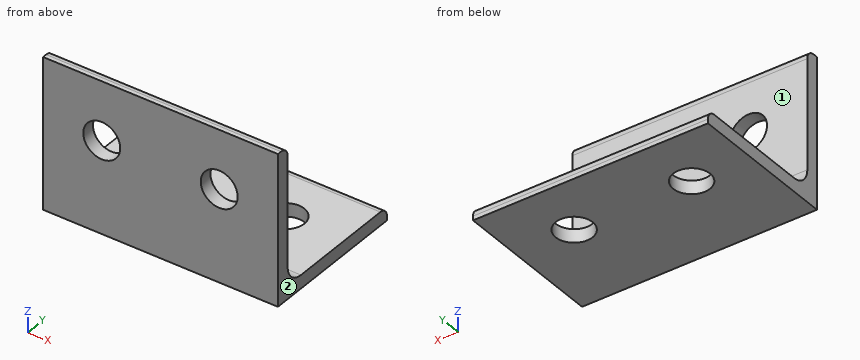
```python
from build123d import *

# Parameters (mm, degrees)
ANGLES_EQUAL_90_X_90_X_8_1_DEPTH = 140
SKETCH12_R                       = 11
CUT_EXTRUDE1_DEPTH               = 190.208879284
LPATTERN1_COUNT                  = 2
LPATTERN1_PITCH                  = 70
CIRPATTERN4_COUNT                = 2
CIRPATTERN4_ANGLE                = 90
CIRPATTERN4_COPY_1_SKETCH_R      = 11
CIRPATTERN4_COPY_1_DEPTH         = 190.208879284


with BuildPart() as part:
    # Sketch11 → Angles equal 90 X 90 X 8(1) (new body)
    with BuildSketch(Plane(origin=(0, 45, 45), x_dir=(0, 1, 0), z_dir=(1, 0, 0))):
        with BuildLine():
            Line((-45, 45), (-45, -45))
            Line((-45, -45), (45, -45))
            Line((45, -45), (45, -42.5))
            ThreePointArc((45, -42.5), (43.389087297, -38.610912703), (39.5, -37))
            Line((39.5, -37), (-26, -37))
            ThreePointArc((-26, -37), (-33.778174593, -33.778174593), (-37, -26))
            Line((-37, -26), (-37, 39.5))
            ThreePointArc((-37, 39.5), (-38.610912703, 43.389087297), (-42.5, 45))
            Line((-42.5, 45), (-45, 45))
        make_face()
    extrude(amount=ANGLES_EQUAL_90_X_90_X_8_1_DEPTH)

    # Sketch12 → Cut-Extrude1 (cut, symmetric)
    with BuildSketch(Plane(origin=(0, 0, 0), x_dir=(1, 0, 0), z_dir=(0, 1, 0))):
        with Locations(Location((35, -55, 0), (0, 0, 90))):
            Circle(SKETCH12_R)
    cut_extrude1 = extrude(amount=CUT_EXTRUDE1_DEPTH, both=True, mode=Mode.SUBTRACT)

    # LPattern1: Cut-Extrude1 ×2
    with Locations(*[(i * LPATTERN1_PITCH, 0, 0) for i in range(1, LPATTERN1_COUNT)]):
        add(cut_extrude1, mode=Mode.SUBTRACT)

    # CirPattern4: Cut-Extrude1 ×2 about axis
    cirpattern4_axis = Axis((-18.99, 0, 0), (-1, 0, 0))
    for i in range(1, CIRPATTERN4_COUNT):
        add(cut_extrude1.rotate(cirpattern4_axis, i * CIRPATTERN4_ANGLE / (CIRPATTERN4_COUNT - 1)), mode=Mode.SUBTRACT)

    # CirPattern4 copy 1 sketch → CirPattern4 copy 1 (cut, symmetric)
    with BuildSketch(Plane(origin=(70, 0, 0), x_dir=(1, 0, 0), z_dir=(0, 0, -1))):
        with Locations(Location((35, -55, 0), (0, 0, 90))):
            Circle(CIRPATTERN4_COPY_1_SKETCH_R)
    extrude(amount=CIRPATTERN4_COPY_1_DEPTH, both=True, mode=Mode.SUBTRACT)


solid = part.part
```
CAD build for the part. Positions are in the model's coordinates, mm. Face numbers are marked on the shaded views. A direction names the side the tool comes from. Round coordinates to 2 decimals unless told otherwise and drop trailing zeros. Order: outer loops, then holes, each group sorted by start corner. A loop starts at its lowest first (then second) coordinate and runs counter-clockwise, first axis right, second up. Notation, with made-up numbers: (-32, 33) - (16, 33) arc R4 ccw to (16, 40) - close; hole circle Ø6 at (73.25, -31.75). An arc over 180 degrees is marked (long way). Answer in a Markdown table with one row per item. Add a question column.
(1) Band-saw the part on B-B on z = 55. List the corners of the cut face in (x, y), and give its area (3 significant figures).
(2) Band-saw the part on D-D on x = 52.5. List the corners of the cut face in (y, z), and give its area (3 significant figures).
(3) Drop flat-ended pins along their axis: pin 1 Ø19.5 at (x, z) = (72.5, 46) entering from +Y; pin 2 Ø1.5 at (x, y) = (52, 38) entering from +Z; pin 3 Ø5 at (x, z) = (125.5, 26.5) entering from -Y. Give the stop position or say it passes through.
(4) Probe L1, parallel to X at y = 4.5, z = 55; L2, parallel to Z at x = 105, y = 2.75; L3, parallel to Y at x = 56, z = 56.5. List the from-to ranges inside material, lowest first. Write a range as [from, to].
(5) 3-axis set-ups, long thin cutter, end or side, ignore diameter. For the marked faces 1 and 2: which of +Z, -Z, +X, -X, +Y, -Y reach the whole face in a straight line?
(6) Band-saw the part on A-A on x = 105. List the corners of the cut face in (y, z), and give its area (3 significant figures).
Data:
| question | item | result |
|---|---|---|
| 1 | outline | (0, 0) - (24, 0) - (24, 8) - (0, 8) - close; (46, 0) - (94, 0) - (94, 8) - (46, 8) - close; (116, 0) - (140, 0) - (140, 8) - (116, 8) - close |
| 1 | area | 768 mm^2 |
| 2 | outline | (0, 0) - (90, 0) - (90, 2.5) arc R5.5 ccw to (84.5, 8) - (19, 8) arc R11 cw to (8, 19) - (8, 84.5) arc R5.5 ccw to (2.5, 90) - (0, 90) - close |
| 2 | area | 1,390 mm^2 |
| 3 | pin 1 | stops at y = 8 |
| 3 | pin 2 | stops at z = 8 |
| 3 | pin 3 | stops at y = 0 |
| 4 | L1 | x = [0, 24], [46, 94], [116, 140] |
| 4 | L2 | z = [0, 44], [66, 89.99] |
| 4 | L3 | y = [0, 8] |
| 5 | face 1 | +Z, +X, -X, +Y |
| 5 | face 2 | +Z, -Z, +X, +Y, -Y |
| 6 | outline | (0, 0) - (44, 0) - (44, 8) - (19, 8) arc R11 cw to (8, 19) - (8, 44) - (0, 44) - close; (0, 66) - (8, 66) - (8, 84.5) arc R5.5 ccw to (2.5, 90) - (0, 90) - close; (66, 0) - (90, 0) - (90, 2.5) arc R5.5 ccw to (84.5, 8) - (66, 8) - close |
| 6 | area | 1,040 mm^2 |
